Read the model definition and answer for the solid it produces. Units are mm, in the model's axes. Face numbers are marked on the shaded views. A direction names the side the tool comes from. Coordinates: 2 decimals unless noted, no trailing zeros. Write each loop counter-clockwise with the first axis right and the second up, starting at its lowest first coordinate (ties: lowest second). Pieces come first, ordered by that corner, then holes.
Item 1: Section A-A (y = -1.75) is taken. Give the vertices of the cut face in (x, z), then the cut area to 3 significant figures.
Item 2: Section C-C (z = -2.58) is taken. Give the vertices of the cut face in (x, y) (3 decimals), then the cut area to 3 significant figures.
Item 3: Section D-D (y = 1.75) is taken. Give the vertices of the cut face in (x, z), then the cut area to 3 significant figures.
Item 4: A tool of negligible diameter and unlimited length cuts with its end or side. For the marked faces 4, 5, 6 and 7, from which of +Z, -Z, +X, -X, +Y, -Y can it reach the whole face along a straight path? Write none if from no direction.
Item 5: Straight lines are drawn through the part: probe 1 along Z at (x, y) = (2.25, 7.25) (3 decimals); probe 2 along Z at (x, y) = (4.04, -3.5); probe 3 along Y at (x, z) = (-6.7, -2.58). For each, find the intervals that lie inside material, in ascending order.
Item 6: Each of these flat-tipped pins is pushed along its axis until it touches: P1, Ø2, axis at x = -5, z = 1, coming from the -Y side; P2, Ø0.7, axis at y = -6.5, z = 0, coming from the -X side; P3, Ø1.4, axis at x = 4, z = -2.5, coming from the +Y side. Where does it stop, or does it pass through?
Item 7: Section B-B (x = 2.75) is taken. Give the vertices of the cut face in (y, z) (3 decimals), then the cut area to 3 significant figures.
Item 8: Determine the mould class of the marked faces 1, 2 and 3 for opening direction Y: released by +Y, released by -Y, zero draft, split by the parting line, or undercut.
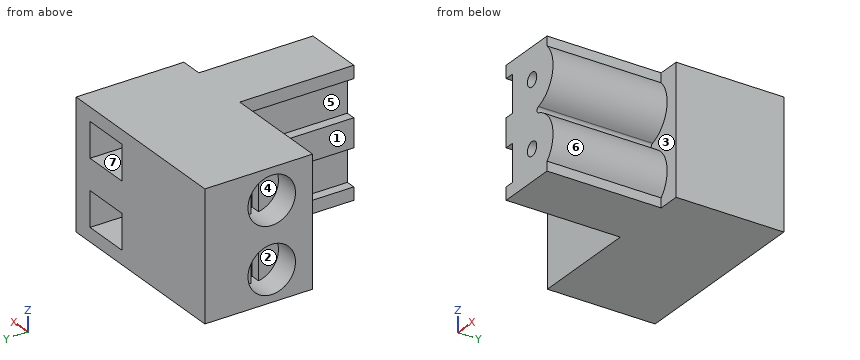
from build123d import *

# Parameters (mm, degrees)
SKETCH1_W           = 15.1
SKETCH1_H           = 10.08
BOSS_EXTRUDE1_DEPTH = 8.5
SKETCH2_R           = 0.55
BOSS_EXTRUDE2_DEPTH = 9
SKETCH3_R           = 1.875
CUT_EXTRUDE1_DEPTH  = 2
CUT_EXTRUDE2_DEPTH  = 2.75
SKETCH4_W           = 3.75
SKETCH4_H           = 2.75
CUT_EXTRUDE3_DEPTH  = 2.9


with BuildPart() as part:
    # Sketch1 → Boss-Extrude1 (new body)
    with BuildSketch(Plane(origin=(0, 0, 0), x_dir=(1, 0, 0), z_dir=(0, 1, 0))):
        Rectangle(SKETCH1_W, SKETCH1_H)
    extrude(amount=BOSS_EXTRUDE1_DEPTH)

    # Sketch2 → Boss-Extrude2 (add)
    with BuildSketch(Plane.XZ):
        with BuildLine():
            Line((5.8, 4.298720454), (5.8, 5.04))
            Line((5.8, 5.04), (1, 5.04))
            Line((1, 5.04), (1, 4.04))
            Line((1, 4.04), (1.75, 4.04))
            Line((1.75, 4.04), (1.75, 1.12))
            Line((1.75, 1.12), (1, 1.12))
            Line((1, 1.12), (1, -1.12))
            Line((1, -1.12), (1.75, -1.12))
            Line((1.75, -1.12), (1.75, -4.04))
            Line((1.75, -4.04), (1, -4.04))
            Line((1, -4.04), (1, -5.04))
            Line((1, -5.04), (5.8, -5.04))
            Line((5.8, -5.04), (5.8, -4.298720454))
            ThreePointArc((5.8, -4.298720454), (6.427646859, -1.987764848), (4.792775244, -0.23800738))
            ThreePointArc((4.792775244, -0.23800738), (4.619276793, 0), (4.792775244, 0.23800738))
            ThreePointArc((4.792775244, 0.23800738), (6.427646859, 1.987764848), (5.8, 4.298720454))
        make_face()
        with Locations((4.04, 2.58)):
            Circle(SKETCH2_R, mode=Mode.SUBTRACT)
        with Locations((4.04, -2.58)):
            Circle(SKETCH2_R, mode=Mode.SUBTRACT)
    extrude(amount=BOSS_EXTRUDE2_DEPTH)

    # Sketch3 → Cut-Extrude1 (cut)
    with BuildSketch(Plane.ZY.offset(7.55)):
        with Locations((-2.58, 3.225)):
            Circle(SKETCH3_R)
        with Locations((2.58, 3.225)):
            Circle(SKETCH3_R)
    extrude(amount=-CUT_EXTRUDE1_DEPTH, mode=Mode.SUBTRACT)

    # Sketch3_3 → Cut-Extrude2 (cut)
    with BuildSketch(Plane.ZY.offset(7.55)):
        with BuildLine():
            Line((-0.729155598, 3.525), (-4.430844402, 3.525))
            ThreePointArc((-4.430844402, 3.525), (-4.455, 3.225), (-4.430844402, 2.925))
            Line((-4.430844402, 2.925), (-0.729155598, 2.925))
            ThreePointArc((-0.729155598, 2.925), (-0.711048656, 3.074514541), (-0.705, 3.225))
            ThreePointArc((-0.705, 3.225), (-0.711048656, 3.375485459), (-0.729155598, 3.525))
        make_face()
        with BuildLine():
            Line((0.729155598, 2.925), (4.430844402, 2.925))
            ThreePointArc((4.430844402, 2.925), (4.448951344, 3.074514541), (4.455, 3.225))
            ThreePointArc((4.455, 3.225), (4.448951344, 3.375485459), (4.430844402, 3.525))
            Line((4.430844402, 3.525), (0.729155598, 3.525))
            ThreePointArc((0.729155598, 3.525), (0.705, 3.225), (0.729155598, 2.925))
        make_face()
    extrude(amount=-CUT_EXTRUDE2_DEPTH, mode=Mode.SUBTRACT)

    # Sketch4 → Cut-Extrude3 (cut)
    with BuildSketch(Plane(origin=(0, 8.5, 0), x_dir=(1, 0, 0), z_dir=(0, 1, 0))):
        with Locations((4.05, -2.58)):
            Rectangle(SKETCH4_W, SKETCH4_H)
        with Locations((4.05, 2.58)):
            Rectangle(SKETCH4_W, SKETCH4_H)
    extrude(amount=-CUT_EXTRUDE3_DEPTH, mode=Mode.SUBTRACT)


solid = part.part
Established:
1. outline: (1, -5.04) - (5.8, -5.04) - (5.8, -4.3) arc R2.46 ccw to (4.79, -0.24) arc R0.25 cw to (4.79, 0.24) arc R2.46 ccw to (5.8, 4.3) - (5.8, 5.04) - (1, 5.04) - (1, 4.04) - (1.75, 4.04) - (1.75, 1.12) - (1, 1.12) - (1, -1.12) - (1.75, -1.12) - (1.75, -4.04) - (1, -4.04) - close; hole circle Ø1.1 at (4.04, -2.58); hole circle Ø1.1 at (4.04, 2.58)
1. area: 44.4 mm2
2. outline: (-7.55, 0) - (1.75, 0) - (1.75, -9) - (3.49, -9) - (3.49, 0) - (4.59, 0) - (4.59, -9) - (6.5, -9) - (6.5, 0) - (7.55, 0) - (7.55, 8.5) - (5.925, 8.5) - (5.925, 5.6) - (2.175, 5.6) - (2.175, 8.5) - (-7.55, 8.5) - (-7.55, 5.1) - (-5.55, 5.1) - (-5.55, 3.525) - (-4.8, 3.525) - (-4.8, 2.925) - (-5.55, 2.925) - (-5.55, 1.35) - (-7.55, 1.35) - close
2. area: 142 mm2
3. outline: (-7.55, -5.04) - (7.55, -5.04) - (7.55, 5.04) - (-7.55, 5.04) - (-7.55, 3.74) - (-5.55, 3.74) - (-5.55, 1.42) - (-7.55, 1.42) - (-7.55, -1.42) - (-5.55, -1.42) - (-5.55, -3.74) - (-7.55, -3.74) - close
3. area: 143 mm2
4. face 4: -X
4. face 5: -X, -Y
4. face 6: +X, -Y
4. face 7: +Y
5. probe 1: z = -5.04 to -3.955, -1.205 to 1.205, 3.955 to 5.04
5. probe 2: z = -5.04 to -3.13, -2.03 to 2.03, 3.13 to 5.04
5. probe 3: y = 0 to 1.35, 5.1 to 8.5
6. P1: stops at y = 0
6. P2: stops at x = 1
6. P3: stops at y = 5.6
7. outline: (-9, -5.04) - (8.5, -5.04) - (8.5, -3.955) - (5.6, -3.955) - (5.6, -1.205) - (8.5, -1.205) - (8.5, 1.205) - (5.6, 1.205) - (5.6, 3.955) - (8.5, 3.955) - (8.5, 5.04) - (-9, 5.04) - close
7. area: 160 mm2
8. face 1: zero draft
8. face 2: undercut
8. face 3: released by -Y
